Check sheet for the modelled part. Datum: model origin and axes. Units: mm. Coordinates: 2 decimals unless noted, no trailing zeros. Write each loop counter-clockwise with the first axis right and the second up, starting at its lowest first coordinate (ties: lowest second). Pieces come first, ordered by that corner, then holes. Notation, with made-up numbers: (45.5, -17.75) -> (91.5, -17.75) arc R26 cw to (91.5, 9.25) -> close; hole circle Ø1 at (54.25, 87). An arc over 180 degrees is marked (long way). One line per item, written item: value. Start each with the question number.
1) Gauge pin test, flat ends, axial feed: P1, Ø1, axis at x = -8, z = -2, coming from the -Y side; P2, Ø13, axis at x = 0, z = 0, coming from the +Y side; P3, Ø1, axis at y = 7.5, z = 8, coming from the -X side; P4, Ø1.5, axis at y = 8.5, z = -3, coming from the +X side. Record the tip position at first contact, or that the pin passes through.
2) Sectioned sample at B-B on y = 4. Enter the section's corners in (x, z), plus the area to 3 significant figures.
3) Draft check along Z on faces 1 (the conical face through (-5.73, 0.24, 9.87)), 2 (the flat face through (2, 3, 5)), 3 (the conical face through (-5.68, 0.24, -9.9)). Enter one of: +Z half, -Z half, draft (parallel to the pull), parting line (faces both ways), or undercut.
4) Sectioned sample at A-A on y = 2.5. Enter the section's corners in (x, z).
5) Scan lines: line 1 along Z through (x, y) = (0, 8); line 2 along Z through (x, y) = (0, 2.05); line 3 along X through (y, z) = (3.5, 6.5). Record each from-to range of solid material in increasing order. Write a range as [from, to].
```python
from build123d import *

# Parameters (mm, degrees)
AUFSATZ_LINEAR_AUSTRAGEN1_DEPTH = 12
SKIZZE2_R                       = 5
SCHNITT_LINEAR_AUSTRAGEN1_DEPTH = 3
M16X1_5_GEWINDEBOHRUNG1_D       = 14.5
M16X1_5_GEWINDEBOHRUNG1_DEPTH   = 9


with BuildPart() as part:
    # Skizze1 → Aufsatz-Linear austragen1 (new body)
    with BuildSketch(Plane(origin=(0, 0, 0), x_dir=(1, 0, 0), z_dir=(0, 1, 0))):
        Polygon((12.701705922, 0), (6.350852961, 11), (-6.350852961, 11), (-12.701705922, 0), (-6.350852961, -11), (6.350852961, -11), align=None)
    extrude(amount=AUFSATZ_LINEAR_AUSTRAGEN1_DEPTH)

    # Skizze2 → Schnitt-Linear austragen1 (cut)
    with BuildSketch(Plane.XZ):
        Circle(SKIZZE2_R)
    extrude(amount=-SCHNITT_LINEAR_AUSTRAGEN1_DEPTH, mode=Mode.SUBTRACT)

    # M16x1.5 Gewindebohrung1
    with Locations(Plane(origin=(0, 12, 0), x_dir=(1, 0, 0), z_dir=(0, 1, 0))):
        with Locations((0, 0)):
            Hole(M16X1_5_GEWINDEBOHRUNG1_D / 2, depth=M16X1_5_GEWINDEBOHRUNG1_DEPTH)

    # Skizze5 → Schnitt-Rotation1 (revolve, cut)
    with BuildSketch(Plane.XY):
        Polygon((-12.701705922, 12), (-11, 12), (-12.701705922, 11.017519628), align=None)
        Polygon((-12.701705922, 0), (-11, 0), (-12.701705922, 0.982480372), align=None)
    revolve(axis=Axis((0, 0, 0), (0, 1, 0)), mode=Mode.SUBTRACT)


solid = part.part
```
Answers:
1. P1: stops at y = 0
1. P2: stops at y = 3
1. P3: stops at x = -8.37
1. P4: stops at x = 11.4
2. outline: (-12.7, 0) -> (-6.35, -11) -> (6.35, -11) -> (12.7, 0) -> (6.35, 11) -> (-6.35, 11) -> close; hole circle Ø14.5 at (0, 0)
2. area: 254 mm2
3. face 1: +Z half
3. face 2: undercut
3. face 3: -Z half
4. outline: (-12.7, 0) -> (-6.35, -11) -> (6.35, -11) -> (12.7, 0) -> (6.35, 11) -> (-6.35, 11) -> close; hole circle Ø10 at (0, 0)
5. line 1: z = [-11, -7.25], [7.25, 11]
5. line 2: z = [-11, -5], [5, 11]
5. line 3: x = [-8.95, -3.21], [3.21, 8.95]
